Autodesk Inventor part; units mm, degrees
ref_plane "YZ Plane" through (0, 0, 0) normal (1, 0, 0) x (0, 1, 0)
ref_plane "XZ Plane" through (0, 0, 0) normal (0, 1, 0) x (-1, 0, 0)
ref_plane "XY Plane" through (0, 0, 0) normal (0, 0, 1) x (1, 0, 0)
sketch "Szkic7" plane through (0, 0, 0) normal (0, 0, 1) x (1, 0, 0)
  circle A0 centre (0, 0) radius 20.955
  dimension "d35" = 41.91
extrude "Wyciągnięcie proste2" add sketch "Szkic7" along normal mid plane 25.8125
chamfer "Faza2" distance 1 angle 45 1 edges at (-20.955, 0, 12.9062)
sketch "Szkic9" plane through (0, 0, 12.9062) normal (0, 0, 1) x (1, 0, 0)
  circle A0 centre (0, 0) radius 19.955
extrude "Wyciągnięcie proste3" add sketch "Szkic9" along normal blind 2.1875
sketch "Szkic10" plane through (0, 0, 15.0938) normal (0, 0, 1) x (1, 0, 0)
  line L0 (-12.9904, 22.5) -> (12.9904, 22.5)
  line L1 (12.9904, 22.5) -> (25.9808, 0)
  line L2 (25.9808, 0) -> (12.9904, -22.5)
  line L3 (12.9904, -22.5) -> (-12.9904, -22.5)
  line L4 (-12.9904, -22.5) -> (-25.9808, 0)
  line L5 (-25.9808, 0) -> (-12.9904, 22.5)
  line L6 (0, 29.337) -> (0, -29.337) construction
  line L7 (-29.337, 0) -> (29.337, 0) construction
  point P0 (0, 0)
  point P1 (0, 0)
  point P2 (0, 22.5)
  dimension "d44" = 45
extrude "Wyciągnięcie proste4" add sketch "Szkic10" along normal blind 7
sketch "Szkic12" plane through (0, 0, 0) normal (0, 1, 0) x (-1, 0, 0)
  line L0 (0, -2.1463) -> (0, 12.8775) construction
  line L1 (-12.9904, 15.0938) -> (-12.9904, 22.0937) construction
  line L2 (-25.9808, 22.0937) -> (-12.9904, 22.0937) construction
  line L3 (-25.9808, 15.0938) -> (-25.9808, 22.0937)
  line L4 (-25.9808, 21.2899) -> (-22.9808, 22.0937)
  line L5 (-25.9808, 22.0937) -> (-12.9904, 22.0937)
  line L6 (-25.9808, 15.0938) -> (-12.9904, 15.0938)
  point P0 (0, 0)
  dimension "d50" = 15
  dimension "d51" = 3
revolve "Obrót2" cut sketch "Szkic12" angle 360 about axis through (0, 0, -10) along (0, 0, 1)
thread "Gwint3"
chamfer "Faza3" distance 1 angle 45 1 edges at (-20.955, 0, -12.9062)
equation "\"d35\" = OD"
equation "\"d36\" = 0.7375 * L"
equation "\"d42\" = 0.0625 * L"
equation "\"d44\" = SW"
equation "\"d45\" = 0.2 * L"
equation "\"d51\" = 0.0666667 * SW"
equation "\"SzerokośćGięciaPodcięcia\" = Grubość"
equation "\"RozmiarPodcięciaNarożnika\" = 4 * Grubość"
equation "\"PromieńPrzejścia\" = PromieńGięcia"
equation "\"Rozmiar_promienia_Jacobiego\" = PromieńGięcia"
equation "\"Wielk_odstępu\" = Grubość"
equation "\"d2\" = PromieńGięcia"
equation "\"d23\" = PromieńGięcia"
equation "\"OD\" = 41.91"
equation "\"SW\" = 45"
equation "\"L\" = 35"
properties part number "Korek sześciokątny BSP 1 1/4'' L=35" material "304"
Could you check a few things on this model? Use its own coordinates, in mm. A direction names the side the tool comes from. Round coordinates to 2 decimals unless told otherwise and drop trailing zeros. Loops run counter-clockwise (first coordinate to the right, second up) from the corner with the lowest first, then second, coordinate; pieces in that order, holes last.
Q1. I want a section at A-A (x = 0). Write out the boundary of the cut face in (y, z) (3 decimals), and give its area (3 significant figures).
Q2. On a 3-axis mill with a long thin cutter (end or side, diameter ignored), from which of +Z, -Z, +X, -X, +Y, -Y can I reach the whole of each face in a straight line? I mean faces 1 (the cylindrical face through (-2.728, -20.777, -0.167)), 2 (the flat face through (0, 0, 22.094)). Say none if no direction works.
Q3. Thinking about a two-plate mould opening in Z: for faces 3 (the flat face through (19.4, 11.4, 18.5)), 4 (the conical face through (-11.825, -20.695, 21.865)), 5 (the cylindrical face through (-15.836, 12.142, 13.985)), 6 (the flat face through (13.4, 15.1, 15.094)), which applies, pulls with the +Z half, pulls with the -Z half, needs draft (parallel to the pull), parting line crosses it, or undercut?
Q4. I want a section at B-B (z = -2). Write out the boundary of the cut face in (x, y) (3 decimals).
Q5. Please list where these lines run through material, in increasing order: L1, parallel to Z at x = -22, y = 4; L2, parallel to Y at x = 7, z = -1; L3, parallel to Y at x = -24, z = 19.
Q6. For P1, Ø10, axis at x = -19.5, z = -1.5, coming from the +Y side; P2, Ø12, axis at y = 7.5, z = 16, coming from the +X side; P3, Ø1, axis at x = -5.5, z = -6, coming from the +Y side, each with a flat end and sliding along its axis, tell me the tip position at first contact or that it passes through.
Answer below:
1. outline: (-22.5, 15.094) - (-19.955, 15.094) - (-19.955, 12.906) - (-20.955, 11.906) - (-20.955, -11.906) - (-19.955, -12.906) - (19.955, -12.906) - (20.955, -11.906) - (20.955, 11.906) - (19.955, 12.906) - (19.955, 15.094) - (22.5, 15.094) - (22.5, 22.094) - (-22.5, 22.094) - close
1. area: 1,480 mm2
2. face 1: -Z
2. face 2: +Z, +X, -X, +Y, -Y
3. face 3: needs draft
3. face 4: pulls with the +Z half
3. face 5: undercut
3. face 6: undercut
4. outline: circle Ø41.91 at (0, 0)
5. L1: z = 15.09 to 22.09
5. L2: y = -19.75 to 19.75
5. L3: y = -3.43 to 3.43
6. P1: stops at y = 15.13
6. P2: stops at x = 25.11
6. P3: stops at y = 20.35
